Here's how the part is built. I have some questions about the finished solid (model axes, mm). A direction names the side the tool comes from. Round coordinates to 2 decimals unless told otherwise and drop trailing zeros. Write each loop counter-clockwise with the first axis right and the second up, starting at its lowest first coordinate (ties: lowest second). Pieces come first, ordered by that corner, then holes. Notation, with made-up numbers: (30.5, 15.5) -> (72.5, 15.5) arc R28 cw to (72.5, 38.5) -> close; hole circle Ø4 at (-35.75, 26.25). An arc over 180 degrees is marked (long way). Answer in a Markdown table with one row per item.
from build123d import *

# Parameters (mm, degrees)
GAP_DEPTH = 103.489078686


with BuildPart() as part:
    # Sketch1 → Base-Revolve (revolve)
    with BuildSketch(Plane.XY, mode=Mode.PRIVATE) as base_revolve_sk:
        Polygon((0, 5.715), (101.6, 5.715), (101.6, 8.89), (97.79, 9.525), (3.81, 9.525), (0, 8.89), align=None)
    revolve(base_revolve_sk.sketch.rotate(Axis((-9.525, 0, 0), (1, 0, 0)), 90), axis=Axis((-9.525, 0, 0), (1, 0, 0)))

    # Sketch2 → Gap (cut, through all)
    with BuildSketch(Plane(origin=(0, 0, 0), x_dir=(0, -1, 0), z_dir=(-1, 0, 0))):
        with BuildLine():
            Line((0, 0), (0.762269345, 9.685550356))
            ThreePointArc((0.762269345, 9.685550356), (0, 9.7155), (-0.762269345, 9.685550356))
            Line((-0.762269345, 9.685550356), (0, 0))
        make_face()
    extrude(amount=-GAP_DEPTH, mode=Mode.SUBTRACT)


solid = part.part
1) We'd pull the mould along Z, two halves only. Please class faces 1 (the face through (50.1, -0.6, 7.6)), 2 (the face through (51.51, -0.24, -5.71)), 3 (the face through (101.6, 0, -6)): +Z half, -Z half, draft (parallel to the pull), parting line (faces both ways), or undercut.
Response:
| item | result |
|---|---|
| face 1 | +Z half |
| face 2 | undercut |
| face 3 | draft |
2) I want a section at B-B, the plane x = 21. List the corners of the cut face in (y, z) for me (3 decimals).
Response:
| item | result |
|---|---|
| outline | (-0.747, 9.496) arc R9.525 ccw (long way) to (0.747, 9.496) -> (0.448, 5.697) arc R5.715 cw (long way) to (-0.448, 5.697) -> close |
3) I need wall thicknesses on line 1 (Y direction, x = 60, z = 0) (3 decimals); line 2 (Z direction, x = 69, y = 0) (3 decimals); line 3 (Z direction, x = 56, y = -4). Which ranges of each line are inside material? Lowest first, please. Write a range as [from, to].
Response:
| item | result |
|---|---|
| line 1 | y = [-9.525, -5.715], [5.715, 9.525] |
| line 2 | z = [-9.525, -5.715] |
| line 3 | z = [-8.64, -4.08], [4.08, 8.64] |
4) Which directions (+Z, -Z, +X, -X, +Y, -Y) give clear straight access to the entire face, cutting with the end or side of a thin tool? Please do faces 4 (the face through (50.1, 0.6, 7.6)), 5 (the face through (50.142, -0.408, -9.516)).
Response:
| item | result |
|---|---|
| face 4 | +Z, +X, -X |
| face 5 | +X, -X |
5) For pin 1 (6 mm diameter, centred on y = -1, z = -7, fed in from -X); pin 2 (4 mm diameter, centred on x = 49, z = 4.5, fed in from +Y); pin 3 (5 mm diameter, centred on x = 87.5, y = 0.5, fed in from +Z); pin 4 (2 mm diameter, centred on x = 11, y = -4.5, fed in from +Z), each with a flat end and sliding along its axis, tell me the tip position at first contact or that it passes through.
Response:
| item | result |
|---|---|
| pin 1 | stops at x = 0 |
| pin 2 | stops at y = 9.19 |
| pin 3 | stops at z = 9.5 |
| pin 4 | stops at z = 8.86 |
6) I want a section at A-A, the plane z = 0. List the corners of the cut face in (x, y) for me (3 decimals), and give its area (3 significant figures).
Response:
| item | result |
|---|---|
| outline | (0, -8.89) -> (3.81, -9.525) -> (97.79, -9.525) -> (101.6, -8.89) -> (101.6, -5.715) -> (0, -5.715) -> close; (0, 5.715) -> (101.6, 5.715) -> (101.6, 8.89) -> (97.79, 9.525) -> (3.81, 9.525) -> (0, 8.89) -> close |
| area | 769 mm^2 |
